Input: part model. Units: mm. Frame: model coordinates. Round coordinates to 2 decimals unless told otherwise and drop trailing zeros. Loops run counter-clockwise (first coordinate to the right, second up) from the corner with the lowest first, then second, coordinate; pieces in that order, holes last. Notation, with made-up numbers: M 23.25,-30.75 L 49.25,-30.75 A19 ccw 49.25,-26.75 Z; hole C -34.75,84.5 d9. An arc over 180 degrees is marked long. Use one line per item in the form item = value. Start each with the question number.
Q1. Section query B-B, the plane y = -70. Output: boundary loops of the cut face in (x, z) (3 decimals), and give its area (3 significant figures).
Q2. Ray query, line 1 along X through (y, z) = (-106, 0.8); line 2 along X through (y, z) = (-109, 1.3); line 3 along Y through (x, z) = (46, 1.35). Return the intervals inside material, ascending.
Q3. First-contact query: P1, Ø3, axis at x = 89.5, y = -38.5, coming from the -Z side; P2, Ø1, axis at y = -42.5, z = 1.5, coming from the +X side. Flat tips, straight axial feed; report the tip coordinate or a pass-through.
Q4. Section query C-C, the plane y = -11. Output: boundary loops of the cut face in (x, z) (3 decimals).
Q5. Section query A-A, the plane z = 1.05. Output: boundary loops of the cut face in (x, y), and give its area (3 significant figures).
```python
from build123d import *

# Parameters (mm, degrees)
BOSS_EXTRUDE1_DEPTH = 3.175


with BuildPart() as part:
    # Sketch1 → Boss-Extrude1 (new body)
    with BuildSketch(Plane.XY):
        with BuildLine():
            Line((0, -6.35), (0, -38.1))
            Line((0, -38.1), (114.3, -152.4))
            Line((114.3, -152.4), (296.8625, -152.4))
            ThreePointArc((296.8625, -152.4), (301.691077882, -150.173995107), (303.134320963, -145.056641147))
            Line((303.134320963, -145.056641147), (281.008014649, -5.356641147))
            ThreePointArc((281.008014649, -5.356641147), (278.860188794, -1.521422118), (274.736193687, 0))
            Line((274.736193687, 0), (6.35, 0))
            ThreePointArc((6.35, 0), (1.859871939, -1.859871939), (0, -6.35))
        make_face()
    extrude(amount=BOSS_EXTRUDE1_DEPTH)


solid = part.part
```
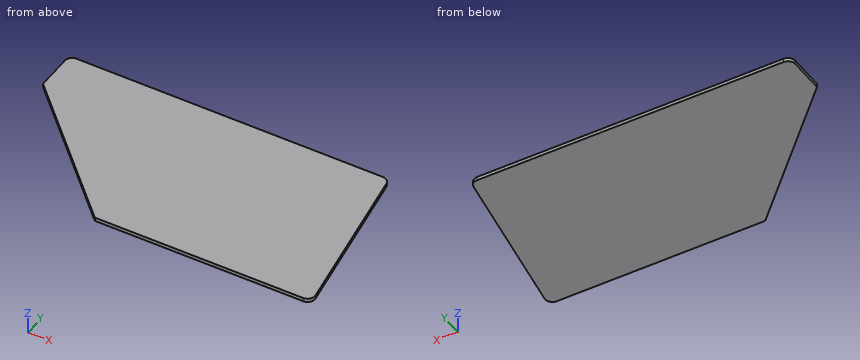
Results found:
q1.outline = M 31.9,0 L 291.247,0 L 291.247,3.175 L 31.9,3.175 Z
q1.area = 823 mm²
q2.line_1 = 67.9 to 296.95
q2.line_2 = 70.9 to 297.42
q2.line_3 = -84.1 to 0
q3.P1 = 0
q3.P2 = 286.97
q4.outline = M 0,0 L 281.902,0 L 281.902,3.175 L 0,3.175 Z
q5.outline = M 0,-38.1 L 114.3,-152.4 L 296.86,-152.4 A6.35 ccw 303.13,-145.06 L 281.01,-5.36 A6.35 ccw 274.74,0 L 6.35,0 A6.35 ccw 0,-6.35 Z
q5.area = 38,000 mm²
